Geometry check sheet. Reference: the model listing, model coordinates, mm. Coordinates: 2 decimals unless noted, no trailing zeros. Write each loop counter-clockwise with the first axis right and the second up, starting at its lowest first coordinate (ties: lowest second). Pieces come first, ordered by that corner, then holes. Notation, with made-up numbers: M 80.25,61 L 97.25,61 A23 cw 97.25,83 Z; hole C -29.75,24.5 d6. An arc over 180 degrees is marked long. Answer as a JSON object with one key per item and string values. Group by question number.
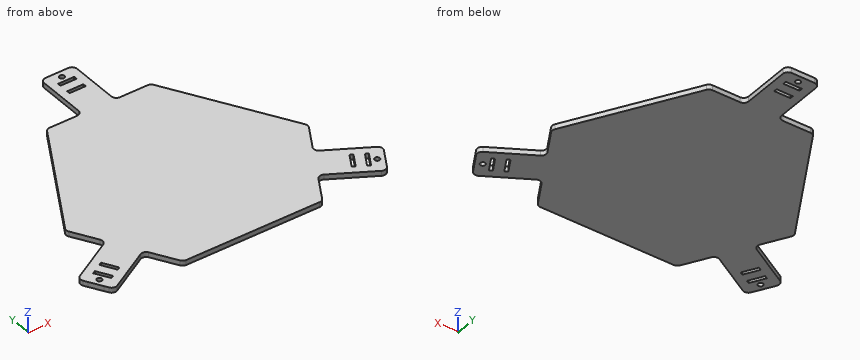
```python
from build123d import *

# Parameters (mm, degrees)
SKETCH_1_R      = 1.5
SKETCH_1_W      = 9.7
SKETCH_1_H      = 1.95
EXTRUDE_3_DEPTH = 3


with BuildPart() as part:
    # Эскиз1 → Бобышка-Вытянуть3 (new body)
    with BuildSketch(Plane.XY):
        with BuildLine():
            Line((-88.837912602, -46.410254038), (-84.611415294, -53.730762114))
            Line((-84.611415294, -53.730762114), (-83.299663948, -56.002782092))
            ThreePointArc((-83.299663948, -56.002782092), (-81.478044872, -57.40055957), (-79.201587737, -57.100858303))
            Line((-79.201587737, -57.100858303), (-54.952876431, -43.100858303))
            ThreePointArc((-54.952876431, -43.100858303), (-52.676419295, -42.801157035), (-50.854800219, -44.198934514))
            Line((-50.854800219, -44.198934514), (-42.598076211, -58.5))
            ThreePointArc((-42.598076211, -58.5), (-41.5, -59.598076211), (-40, -60))
            Line((-40, -60), (40, -60))
            ThreePointArc((40, -60), (41.5, -59.598076211), (42.598076211, -58.5))
            Line((42.598076211, -58.5), (50.854800219, -44.198934514))
            ThreePointArc((50.854800219, -44.198934514), (52.676419295, -42.801157035), (54.952876431, -43.100858303))
            Line((54.952876431, -43.100858303), (79.201587737, -57.100858303))
            ThreePointArc((79.201587737, -57.100858303), (81.478044872, -57.40055957), (83.299663948, -56.002782092))
            Line((83.299663948, -56.002782092), (84.611415294, -53.730762114))
            Line((84.611415294, -53.730762114), (88.837912602, -46.410254038))
            Line((88.837912602, -46.410254038), (90.149663948, -44.13823406))
            ThreePointArc((90.149663948, -44.13823406), (90.449365215, -41.861776924), (89.051587737, -40.040157848))
            Line((89.051587737, -40.040157848), (64.802876431, -26.040157848))
            ThreePointArc((64.802876431, -26.040157848), (63.405098952, -24.218538772), (63.704800219, -21.942081637))
            Line((63.704800219, -21.942081637), (71.961524227, -7.641016151))
            ThreePointArc((71.961524227, -7.641016151), (72.363448016, -6.141016151), (71.961524227, -4.641016151))
            Line((71.961524227, -4.641016151), (31.961524227, 64.641016151))
            ThreePointArc((31.961524227, 64.641016151), (30.863448016, 65.739092363), (29.363448016, 66.141016151))
            Line((29.363448016, 66.141016151), (12.85, 66.141016151))
            ThreePointArc((12.85, 66.141016151), (10.728679656, 67.019695808), (9.85, 69.141016151))
            Line((9.85, 69.141016151), (9.85, 97.141016151))
            ThreePointArc((9.85, 97.141016151), (8.971320344, 99.262336495), (6.85, 100.141016151))
            Line((6.85, 100.141016151), (4.226497308, 100.141016151))
            Line((4.226497308, 100.141016151), (-4.226497308, 100.141016151))
            Line((-4.226497308, 100.141016151), (-6.85, 100.141016151))
            ThreePointArc((-6.85, 100.141016151), (-8.971320344, 99.262336495), (-9.85, 97.141016151))
            Line((-9.85, 97.141016151), (-9.85, 69.141016151))
            ThreePointArc((-9.85, 69.141016151), (-10.728679656, 67.019695808), (-12.85, 66.141016151))
            Line((-12.85, 66.141016151), (-29.363448016, 66.141016151))
            ThreePointArc((-29.363448016, 66.141016151), (-30.863448016, 65.739092363), (-31.961524227, 64.641016151))
            Line((-31.961524227, 64.641016151), (-71.961524227, -4.641016151))
            ThreePointArc((-71.961524227, -4.641016151), (-72.363448016, -6.141016151), (-71.961524227, -7.641016151))
            Line((-71.961524227, -7.641016151), (-63.704800219, -21.942081637))
            ThreePointArc((-63.704800219, -21.942081637), (-63.405098952, -24.218538772), (-64.802876431, -26.040157848))
            Line((-64.802876431, -26.040157848), (-89.051587737, -40.040157848))
            ThreePointArc((-89.051587737, -40.040157848), (-90.449365215, -41.861776924), (-90.149663948, -44.13823406))
            Line((-90.149663948, -44.13823406), (-88.837912602, -46.410254038))
        make_face()
        with Locations((-83.260562333, -48.070508076)):
            Circle(SKETCH_1_R, mode=Mode.SUBTRACT)
        with Locations(Location((83.260562333, -48.070508076, 0), (0, 0, 180))):
            Circle(SKETCH_1_R, mode=Mode.SUBTRACT)
        with Locations((0, 96.141016151)):
            Circle(SKETCH_1_R, mode=Mode.SUBTRACT)
        Polygon((-77.804473419, -50.520731284), (-82.654473419, -42.120284867), (-80.965723882, -41.145284867), (-76.115723882, -49.545731284), align=None, mode=Mode.SUBTRACT)
        Polygon((-71.309282891, -46.770731284), (-76.159282891, -38.370284867), (-74.470533354, -37.395284867), (-69.620533354, -45.795731284), align=None, mode=Mode.SUBTRACT)
        Polygon((69.620533354, -45.795731284), (74.470533354, -37.395284867), (76.159282891, -38.370284867), (71.309282891, -46.770731284), align=None, mode=Mode.SUBTRACT)
        Polygon((76.115723882, -49.545731284), (80.965723882, -41.145284867), (82.654473419, -42.120284867), (77.804473419, -50.520731284), align=None, mode=Mode.SUBTRACT)
        with Locations((0, 91.666016151)):
            Rectangle(SKETCH_1_W, SKETCH_1_H, mode=Mode.SUBTRACT)
        with Locations((0, 84.166016151)):
            Rectangle(SKETCH_1_W, SKETCH_1_H, mode=Mode.SUBTRACT)
    extrude(amount=EXTRUDE_3_DEPTH)


solid = part.part
```
1) Section check B-B (z = 0.9). State how many separate pieces and enclosed holes the cut face has, then the cut area to 3 significant figures.
2) Section check A-A (x = -27). Record the cut outline in (y, z), then the cut area to 3 significant figures.
3) Material ranges on probe 1 along Y at (x, z) = (-82, 1.05); probe 2 along Y at (x, z) = (71.5, 1.3); probe 3 along X at (y, z) = (72.5, 1.85), recorded low to high. Write a range as [from, to].
4) Section check C-C (y = 47.5). Record the cut outline in (x, z).
5) Go/stop test with flat-tipped pins: pin 1 Ø1.5 at (x, z) = (-20.5, 1.5) entering from +Y; pin 2 Ø1.5 at (x, z) = (53.5, 1.5) entering from -Y; pin 3 Ø0.6 at (y, z) = (84, 1) entering from +X. Record where each tip stops, or that it passes through.
Entries:
{
 "1": {"separate pieces": "1", "enclosed holes": "9", "area": "15,600 mm^2"},
 "2": {"outline": "M -60,0 L 66.14,0 L 66.14,3 L -60,3 Z", "area": "378 mm^2"},
 "3": {"probe 1": "[-57.21, -48.88], [-47.26, -43.25], [-41.74, -35.97]", "probe 2": "[-52.65, -46.44], [-42.54, -29.91], [-8.44, -3.84]", "probe 3": "[-9.85, 9.85]"},
 "4": {"outline": "M -41.86,0 L 41.86,0 L 41.86,3 L -41.86,3 Z"},
 "5": {"pin 1": "y = 66.14", "pin 2": "y = -42.81", "pin 3": "x = 9.85"}
}
